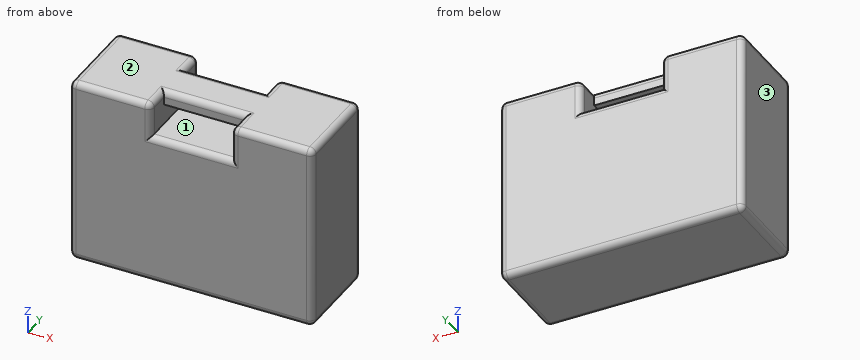
```python
from build123d import *

# Parameters (mm, degrees)
F0_W     = 390
F0_H     = 300
F0_W_2   = 129.2868405581
F0_H_2   = 32.5715690851
F1_DEPTH = 72.5
F2_W     = 129.2868405581
F2_H     = 22.3345696926
F3_DEPTH = 40
F4_R     = 10


# Not quite as in the source:
# - a pattern or mirror of a feature is missing from the dataset's text; its kind, count and spacing are read off the source's solid


with BuildPart() as f1:
    # F0 (on Front) → F1 (new body, symmetric)
    with BuildSketch(Plane.XZ):
        Rectangle(F0_W, F0_H)
        with Locations((0, 111.3796457648)):
            Rectangle(F0_W_2, F0_H_2, mode=Mode.SUBTRACT)
    extrude(amount=F1_DEPTH, both=True)

    # F2 (on face) → F3 (cut)
    with BuildSketch(Plane.XZ.offset(72.5)):
        with Locations((0, 138.8327151537)):
            Rectangle(F2_W, F2_H)
    f3 = extrude(amount=-F3_DEPTH, mode=Mode.SUBTRACT)

    # F3_copies: F3 across plane
    add(f3.mirror(Plane.ZX), mode=Mode.SUBTRACT)

    # F4
    f4_edges = [f1.edges().sort_by_distance(p)[0] for p in [
        (0, -72.5, -150),
        (195, -72.5, 0),
        (129.82171, -72.5, 150),
        (64.64342, -72.5, 122.546931),
        (0, -72.5, 95.093861),
        (-64.64342, -72.5, 122.546931),
        (-129.82171, -72.5, 150),
        (-195, -72.5, 0),
        (-195, 0, 150),
        (-195, 72.5, 0),
        (-195, 0, -150),
        (195, 0, 150),
        (64.64342, -52.5, 150),
        (0, -32.5, 150),
        (-64.64342, -52.5, 150),
        (-129.82171, 72.5, 150),
        (-64.64342, 52.5, 150),
        (0, 32.5, 150),
        (64.64342, 52.5, 150),
        (129.82171, 72.5, 150),
        (0, 72.5, -150),
        (195, 72.5, 0),
        (64.64342, 72.5, 122.546931),
        (0, 72.5, 95.093861),
        (-64.64342, 72.5, 122.546931),
        (195, 0, -150),
    ]]
    fillet(f4_edges, radius=F4_R)


solid = f1.part
```
Source: CAD feature listing. Evaluate the final solid. Frame: model axes, mm. Face numbers are marked on the shaded views. Coordinates: 2 decimals unless noted, no trailing zeros. Loops run counter-clockwise (first coordinate to the right, second up) from the corner with the lowest first, then second, coordinate; pieces in that order, holes last. Notation, with made-up numbers: (38.5, 59.5) - (83.5, 59.5) arc R8 ccw to (83.5, 74.5) - close; hole circle Ø6 at (27, 23.25). An arc over 180 degrees is marked (long way). Answer as CSV lines item,"result".
1. Ray query, line 1 (Z direction, x = -34.5, y = -20.5); line 2 (X direction, y = 13, z = 96.5); line 3 (Z direction, x = -12, y = -51.5). Return the intervals inside material, ascending.
Established:
line 1,"z = -150 to 95.09, 127.67 to 150"
line 2,"x = -195 to -64.64, 64.64 to 195"
line 3,"z = -150 to 95.09"
2. Mould query, pull axis Z, two halves, no side actions, for the marked faces 1, 2 and 3. Classes: released by +Z, released by -Z, zero draft, split by the parting line, or undercut.
Established:
face 1,"undercut"
face 2,"released by +Z"
face 3,"zero draft"
3. Contact query for flat-ended pins moving along their axis: pin 1 (13.5 mm diameter, centred on x = -17.5, z = 131.5, fed in from -Y); pin 2 (13.5 mm diameter, centred on x = -17.5, z = 131.5, fed in from +Y). Output: stop coordinate, or through.
Established:
pin 1,"stops at y = -32.5"
pin 2,"stops at y = 32.5"
4. Section A-A (y = 5.5). Return loops of the section in (x, z).
Established:
outline,"(-195, -140) arc R10 ccw to (-185, -150) - (185, -150) arc R10 ccw to (195, -140) - (195, 140) arc R10 ccw to (185, 150) - (-185, 150) arc R10 ccw to (-195, 140) - close; hole (-64.64, 95.09) - (64.64, 95.09) - (64.64, 127.67) - (-64.64, 127.67) - close"
5. Section C-C (x = 30.5). Return loops of the section in (y, z).
Established:
outline,"(-72.5, -140) arc R10 ccw to (-62.5, -150) - (62.5, -150) arc R10 ccw to (72.5, -140) - (72.5, 85.09) arc R10 ccw to (62.5, 95.09) - (-62.5, 95.09) arc R10 ccw to (-72.5, 85.09) - close; (-32.5, 127.67) - (32.5, 127.67) - (32.5, 140) arc R10 ccw to (22.5, 150) - (-22.5, 150) arc R10 ccw to (-32.5, 140) - close"
6. Section B-B (z = 122). Return loops of the section in (x, y), then the cut area to 3 significant figures.
Established:
outline,"(-195, -62.5) arc R10 ccw to (-185, -72.5) - (-74.64, -72.5) arc R10 ccw to (-64.64, -62.5) - (-64.64, 62.5) arc R10 ccw to (-74.64, 72.5) - (-185, 72.5) arc R10 ccw to (-195, 62.5) - close; (64.64, -62.5) arc R10 ccw to (74.64, -72.5) - (185, -72.5) arc R10 ccw to (195, -62.5) - (195, 62.5) arc R10 ccw to (185, 72.5) - (74.64, 72.5) arc R10 ccw to (64.64, 62.5) - close"
area,"37,600 mm2"
